```python
from build123d import *

# Parameters (mm, degrees)
F1_DEPTH  = 40
F2_R      = 8.25
F3_DEPTH  = 5
F4_W      = 5
F4_H      = 55
F4_W_2    = 40
F5_DEPTH  = 16.3
F6_W      = 7
F6_H      = 39
F7_DEPTH  = 55.001
F8_SIZE   = 10
F9_R      = 2.5
F10_DEPTH = 66.401
F11_W     = 30
F11_H     = 10
F12_DEPTH = 50
F13_W     = 30
F13_H     = 10
F14_DEPTH = 50
F15_SIZE  = 1.5
F16_R     = 5
F17_R     = 2.5
F18_DEPTH = 2.5
F19_R     = 2.49999
F20_R     = 2


# Not quite as in the source:
# - a fillet or chamfer is up to 0.001 mm smaller than in the source, because OpenCascade refuses the exact size
# - a feature names something its author has since deleted; it is built from what else it names


with BuildPart() as f1:
    # F0 (on Front) → F1 (new body)
    with BuildSketch(Plane.XZ):
        Polygon((0, 55), (0, 0), (50.1, 0), (50.1, 5), (0.1, 5), (0.1, 50), (50.1, 50), (50.1, 55), align=None)
    extrude(amount=-F1_DEPTH)

    # F2 (on face) → F3 (cut, through all)
    with BuildSketch(Plane.XY.offset(55)):
        with Locations((35, 20)):
            Circle(F2_R)
    extrude(amount=-F3_DEPTH, mode=Mode.SUBTRACT)

    # F4 (on face) → F5 (join)
    with BuildSketch(Plane(origin=(0, 0, 0), x_dir=(0, -1, 0), z_dir=(-1, 0, 0))):
        with Locations((2.5, 27.5)):
            Rectangle(F4_W, F4_H)
        with Locations((-20, 27.5)):
            Rectangle(F4_W_2, F4_H)
        with Locations((-42.5, 27.5)):
            Rectangle(F4_W, F4_H)
    extrude(amount=F5_DEPTH)

    # F6 (on face) → F7 (cut, through all)
    with BuildSketch(Plane(origin=(0, 0, 0), x_dir=(1, 0, 0), z_dir=(0, 0, -1))):
        with Locations((-8.15, -20)):
            Rectangle(F6_W, F6_H)
    extrude(amount=-F7_DEPTH, mode=Mode.SUBTRACT)

    # F8
    f8_edges = [f1.edges().sort_by_distance(p)[0] for p in [
        (0.1, 20, 5),
        (0.1, 20, 50),
    ]]
    chamfer(f8_edges, length=F8_SIZE)

    # F9 (on face) → F10 (cut, through all)
    with BuildSketch(Plane(origin=(-16.3, 0, 0), x_dir=(0, -1, 0), z_dir=(-1, 0, 0))):
        with Locations((-20, 15)):
            Circle(F9_R)
        with Locations((-20, 40)):
            Circle(F9_R)
    extrude(amount=-F10_DEPTH, mode=Mode.SUBTRACT)

    # F11 (on face) → F12 (cut)
    with BuildSketch(Plane.YZ.offset(50.1)):
        with Locations((20, 10)):
            Rectangle(F11_W, F11_H)
    extrude(amount=-F12_DEPTH, mode=Mode.SUBTRACT)

    # F13 (on face) → F14 (cut)
    with BuildSketch(Plane.YZ.offset(50.1)):
        with Locations((20, 45)):
            Rectangle(F13_W, F13_H)
    extrude(amount=-F14_DEPTH, mode=Mode.SUBTRACT)

    # F15
    f15_edges = [f1.edges().sort_by_distance(p)[0] for p in [
        (-11.65, 20, 55),
        (-8.15, 39.5, 55),
        (-4.65, 20, 55),
        (-8.15, 0.5, 55),
        (-11.65, 20, 0),
        (-8.15, 0.5, 0),
        (-4.65, 20, 0),
        (-8.15, 39.5, 0),
    ]]
    chamfer(f15_edges, length=F15_SIZE)

    # F16
    f16_edges = [f1.edges().sort_by_distance(p)[0] for p in [
        (50.1, 0, 52.5),
        (50.1, 40, 52.5),
        (50.1, 40, 2.5),
        (50.1, 0, 2.5),
        (0.1, 37.5, 15),
        (0.1, 2.5, 15),
        (10.1, 2.5, 5),
        (10.1, 37.5, 5),
        (0.1, 2.5, 40),
        (0.1, 37.5, 40),
        (10.1, 37.5, 50),
        (10.1, 2.5, 50),
    ]]
    fillet(f16_edges, radius=F16_R)

    # F17 (on face) → F18 (join)
    with BuildSketch(Plane.XY.offset(5)):
        with Locations((35.1, 5)):
            Circle(F17_R)
        with Locations((35.1, 35)):
            Circle(F17_R)
    extrude(amount=F18_DEPTH)

    # F19 (radius 2.5 in the source; OpenCascade refuses exactly that, so slightly less here)
    f19_edges = [f1.edges().sort_by_distance(p)[0] for p in [
        (32.6, 5, 7.5),
        (32.6, 35, 7.5),
    ]]
    fillet(f19_edges, radius=F19_R)

    # F20
    f20_edges = [f1.edges().sort_by_distance(p)[0] for p in [
        (-8.15, -5, 0),
        (-8.15, 45, 0),
        (-16.3, 20, 0),
        (22.55, 40, 0),
    ]]
    fillet(f20_edges, radius=F20_R)


solid = f1.part
```
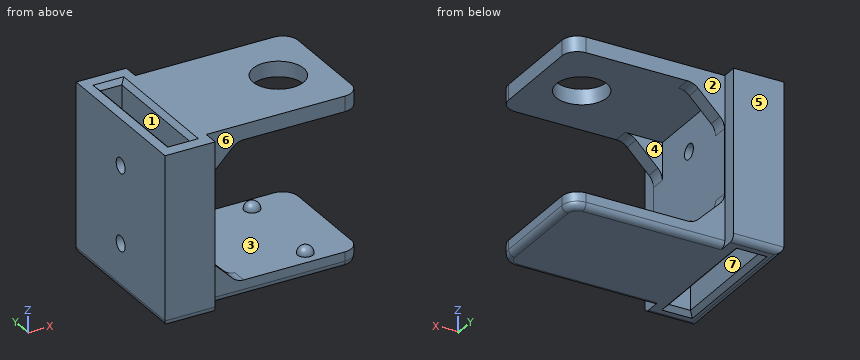
Here's how the part is built. I have some questions about the finished solid (model axes, mm). Face numbers are marked on the shaded views. A direction names the side the tool comes from. Coordinates: 2 decimals unless noted, no trailing zeros. Loops run counter-clockwise (first coordinate to the right, second up) from the corner with the lowest first, then second, coordinate; pieces in that order, holes last. Notation, with made-up numbers: (65, 24) - (69, 24) arc R14 ccw to (69, 37) - close; hole circle Ø1 at (-9.75, 1). An arc over 180 degrees is marked (long way). Return JSON: item names as keys, results as strings. Group by question number.
Item 1: I need wall thicknesses on line 1 (Z direction, x = -14.5, y = 20); line 2 (Y direction, x = -11, z = 19); line 3 (X direction, y = 23, z = 28.5). Which ranges of each line are inside material? Lowest first, please. Write a range as from..to.
Item 2: Will these pins go through, and if not, where does the flat tip stop? P1, Ø9.5, axis at x = 8.5, z = 10.5, coming from the -Y side; P2, Ø8, axis at y = 2.5, z = 20.5, coming from the +X side; P3, Ø3, axis at y = 20, z = 15, coming from the +X side (1 decimal); P4, Ø13.5, axis at x = 7, z = 12, coming from the +Y side.
Item 3: If we section it at B-B on x = -6.5: Write out the boundary of the cut face in (y, z).
Item 4: If we section it at D-D on y = 20: State how many separate pieces and enclosed holes the cut face has, and give its area (3 significant figures).
Item 5: If we section it at C-C on z = 33.5: Write out the boundary of the cut face in (x, y).
Item 6: On a 3-axis mill with a long thin cutter (end or side, diameter ignored), from which of +Z, -Z, +X, -X, +Y, -Y can I reach the whole of each face in a straight line? I mean the marked faces 1, 2, 3 and 4. Say none if no direction works.
Item 7: If we section it at A-A on z = 9: Write out the boundary of the cut face in (x, y).
Item 8: We'd pull the mould along Y, two halves only. Please class the marked faces 5, 6 and 7: +Y half, -Y half, draft (parallel to the pull), parting line (faces both ways), or undercut.
Calculated:
{
 "1": {"line 1": "z = 0.01..12.5, 17.5..37.5, 42.5..55", "line 2": "y = -5..0.5, 39.5..45", "line 3": "x = -16.3..-11.65, -4.65..0.1"},
 "2": {"P1": "stops at y = 0", "P2": "stops at x = 0.13", "P3": "passes through", "P4": "stops at y = 40"},
 "3": {"outline": "(-5, 2) arc R2 ccw to (-3, 0) - (-1, 0) - (0.5, 1.5) - (0.5, 53.5) - (-1, 55) - (-5, 55) - close; (39.5, 1.5) - (41, 0) - (43, 0) arc R2 ccw to (45, 2) - (45, 55) - (41, 55) - (39.5, 53.5) - close"},
 "4": {"separate pieces": "7", "enclosed holes": "0", "area": "834 mm^2"},
 "5": {"outline": "(-16.3, -5) - (0, -5) - (0, 0) - (0.1, 0) - (0.1, 40) - (0, 40) - (0, 45) - (-16.3, 45) - close; hole (-11.65, 0.5) - (-4.65, 0.5) - (-4.65, 39.5) - (-11.65, 39.5) - close"},
 "6": {"face 1": "+Z, -Z", "face 2": "+Z, -Z, +X, +Y", "face 3": "none", "face 4": "+X"},
 "7": {"outline": "(-16.3, -5) - (0, -5) - (0, 0) - (6.1, 0) - (6.1, 5) - (0.1, 5) - (0.1, 35) - (6.1, 35) - (6.1, 40) - (0, 40) - (0, 45) - (-16.3, 45) - close; hole (-11.65, 0.5) - (-4.65, 0.5) - (-4.65, 39.5) - (-11.65, 39.5) - close"},
 "8": {"face 5": "+Y half", "face 6": "-Y half", "face 7": "undercut"}
}
